The model under review builds one solid part; all positions refer to its coordinate system, in mm. A direction names the side the tool comes from. Round coordinates to 2 decimals unless told otherwise and drop trailing zeros. Order: outer loops, then holes, each group sorted by start corner. A loop starts at its lowest first (then second) coordinate and runs counter-clockwise, first axis right, second up.
1) Consider section B-B (x = 4.5). Give the boundary of the cut face in (y, z), then the cut area to 3 significant figures.
2) Consider section C-C (y = 2). Give the boundary of the cut face in (x, z), then the cut area to 3 significant figures.
3) Consider section D-D (x = 2). Give the boundary of the cut face in (y, z).
4) Consider section A-A (z = 1.5). Give the boundary of the cut face in (x, y), then the cut area to 3 significant figures.
5) To check wall thickness, follow L1, parallel to Y at x = 11, z = 3; L2, parallel to X at y = 4.75, z = -16.5; L3, parallel to Y at x = 8, z = -1. State the ranges of each line that lie inside material, in increasing order.
6) Machinability: for faces 4 (the face through (13, 2, 12)), 5 (the face through (11.5, 2.07, 9.97)), 6 (the face through (7.9, 2.5, 5)), which of the approach directions +Z, -Z, +X, -X, +Y, -Y give a long, thin tool a straight path to every point of the face, cutting with its end or side? Answer none if there is none.
7) Clearance check with flat-ended pins moving along their axes: P1, Ø5, axis at x = 4.5, z = -10, coming from the -Y side; P2, Ø1.5, axis at x = 4, y = 5, coming from the -Z side; P3, Ø1.5, axis at y = 5, z = -13, coming from the +X side. State where each tip first meets the part, or that it passes through.
8) Mouldability with a two-part tool opening along X and no side actions: class faces 1 (the face through (16, 5, 4)), 2 (the face through (1.675, 5.536, 9.972)), 3 (the face through (8, 0, 4)) as pulls with the +X half, pulls with the -X half, needs draft (parallel to the pull), parting line crosses it, or undercut.
from build123d import *

# Parameters (mm, degrees)
F0_W     = 16
F0_H     = 10
F1_DEPTH = 8
F2_R     = 1.5
F3_DEPTH = 4
F4_W     = 12.605189
F4_H     = 7.011637
F5_DEPTH = 5
F6_R     = 2.097092
F6_R_2   = 1.192292
F7_DEPTH = 25


with BuildPart() as f1:
    # F0 (on Top) → F1 (new body)
    with BuildSketch(Plane.XY):
        with Locations((8, 5)):
            Rectangle(F0_W, F0_H)
    extrude(amount=F1_DEPTH)

    # F2 (on face) → F3 (join)
    with BuildSketch(Plane.XY.offset(8)):
        with Locations((2, 2)):
            Circle(F2_R)
        with Locations((13, 2)):
            Circle(F2_R)
        with Locations((13, 7)):
            Circle(F2_R)
        with Locations((2, 7)):
            Circle(F2_R)
    extrude(amount=F3_DEPTH)

    # F4 (on face) → F5 (cut)
    with BuildSketch(Plane(origin=(0, 0, 0), x_dir=(1, 0, 0), z_dir=(0, 0, -1))):
        with Locations((7.999999, -4.921217)):
            Rectangle(F4_W, F4_H)
    extrude(amount=-F5_DEPTH, mode=Mode.SUBTRACT)

    # F6 (on face) → F7 (join)
    with BuildSketch(Plane(origin=(0, 0, 5), x_dir=(1, 0, 0), z_dir=(0, 0, -1))):
        with Locations((7.887701, -4.859625)):
            Circle(F6_R)
        with Locations((7.887701, -4.859625)):
            Circle(F6_R_2, mode=Mode.SUBTRACT)
    extrude(amount=F7_DEPTH)


solid = f1.part
Answer below:
1. outline: (0, 0) - (1.42, 0) - (1.42, 5) - (8.43, 5) - (8.43, 0) - (10, 0) - (10, 8) - (0, 8) - close
1. area: 44.9 mm2
2. outline: (0, 0) - (1.7, 0) - (1.7, 5) - (14.3, 5) - (14.3, 0) - (16, 0) - (16, 8) - (14.5, 8) - (14.5, 12) - (11.5, 12) - (11.5, 8) - (3.5, 8) - (3.5, 12) - (0.5, 12) - (0.5, 8) - (0, 8) - close
2. area: 89.0 mm2
3. outline: (0, 0) - (1.42, 0) - (1.42, 5) - (8.43, 5) - (8.43, 0) - (10, 0) - (10, 8) - (8.5, 8) - (8.5, 12) - (5.5, 12) - (5.5, 8) - (3.5, 8) - (3.5, 12) - (0.5, 12) - (0.5, 8) - (0, 8) - close
4. outline: (0, 0) - (16, 0) - (16, 10) - (0, 10) - close; circle Ø4.19 at (7.89, 4.86); hole (1.7, 1.42) - (14.3, 1.42) - (14.3, 8.43) - (1.7, 8.43) - close; hole circle Ø2.38 at (7.89, 4.86)
4. area: 81.0 mm2
5. L1: y = 0 to 1.42, 8.43 to 10
5. L2: x = 5.79 to 6.7, 9.07 to 9.98
5. L3: y = 2.77 to 3.67, 6.05 to 6.95
6. face 4: +Z, +X, -X, +Y, -Y
6. face 5: +Z
6. face 6: -Z
7. P1: stops at y = 2.96
7. P2: stops at z = 5
7. P3: stops at x = 9.98
8. face 1: pulls with the +X half
8. face 2: undercut
8. face 3: needs draft
